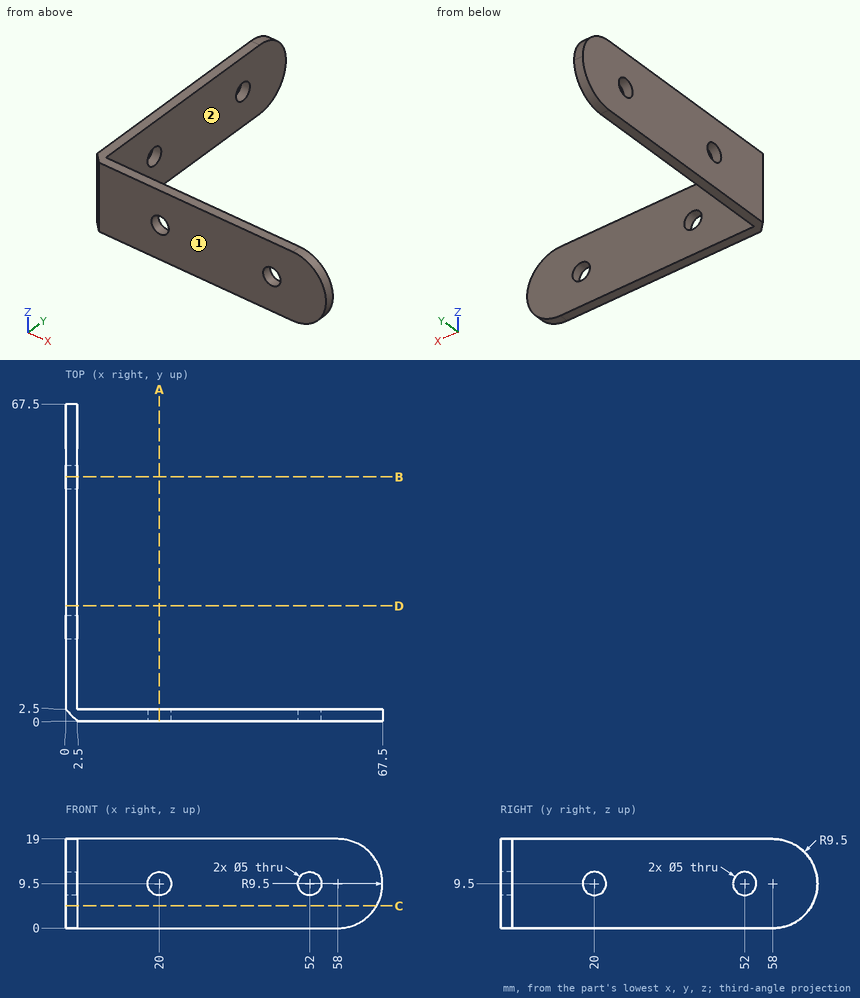
Verification items for this drawing (mm, ordinates from the low corner). A direction names the side the tool comes from. Give positions to 0.01 mm unless a question says otherwise; leave off trailing zeros. Order: outer loops, then holes, each group sorted by start corner. A loop starts at its lowest first (then second) coordinate and runs counter-clockwise, first axis right, second up. Notation, with made-up numbers: M 67.25,2.25 L 114.25,2.25 A18 cw 114.25,24.25 Z; hole C 31,-8.75 d3. An arc over 180 degrees is marked long. Use a Markdown table: item, result.
Item 1: Section check C-C (z = 4.75). Record the cut outline in (x, y), and give its area (3 significant figures).
Answers follow:
| item | result |
|---|---|
| outline | M 0,2.5 L 2.5,0 L 66.23,0 L 66.23,2.5 L 2.5,2.5 L 2.5,66.23 L 0,66.23 Z |
| area | 322 mm2 |
Item 2: Section check D-D (y = 24.5). Record the cut outline in (x, z).
Answers follow:
| item | result |
|---|---|
| outline | M 0,0 L 2.5,0 L 2.5,19 L 0,19 Z |
Item 3: Depth check by flat-ended pin: P1, Ø6, axis at x = 19.5, z = 13.5, coming from the +Y side; P2, Ø6, axis at y = 52, z = 9.5, coming from the +X side. Enter the tip coordinate at first touch or a pass-through.
Answers follow:
| item | result |
|---|---|
| P1 | stops at y = 2.5 |
| P2 | stops at x = 2.5 |
Item 4: Material ranges on line 1 along Z through (x, y) = (52, 0.65); line 2 along Y through (x, z) = (1.8, 9.5); line 3 along Y through (x, z) = (59, 15), recorded low to high.
Answers follow:
| item | result |
|---|---|
| line 1 | z = 0 to 7, 12 to 19 |
| line 2 | y = 0.7 to 17.5, 22.5 to 49.5, 54.5 to 67.5 |
| line 3 | y = 0 to 2.5 |
Item 5: Tool access check on the marked faces 1 and 2. Record the directions out of +Z, -Z, +X, -X, +Y, -Y that give a thin tool (end or side, any length) a straight path to the whole face; none if there is none.
Answers follow:
| item | result |
|---|---|
| face 1 | +Z, -Z, +X, -X, -Y |
| face 2 | +Z, -Z, +X, +Y |
Item 6: Section check A-A (x = 20). Record the cut outline in (y, z).
Answers follow:
| item | result |
|---|---|
| outline | M 0,0 L 2.5,0 L 2.5,7 L 0,7 Z; M 0,12 L 2.5,12 L 2.5,19 L 0,19 Z |
